from build123d import *

# Parameters (mm, degrees)
SKETCH1_R                                           = 8.5
BOSS_EXTRUDE1_DEPTH                                 = 33.5
SKETCH2_W                                           = 53
SKETCH2_H                                           = 50
CUT_EXTRUDE1_DEPTH                                  = 30
SKETCH3_W                                           = 53
SKETCH3_H                                           = 10
BOSS_EXTRUDE2_DEPTH                                 = 13
FILLET1_R                                           = 15
CSK_FOR_M4_COUNTERSUNK_FLAT_HEAD_SCREW1_D           = 4.3
CSK_FOR_M4_COUNTERSUNK_FLAT_HEAD_SCREW1_CSINK_D     = 9.4
CSK_FOR_M4_COUNTERSUNK_FLAT_HEAD_SCREW1_CSINK_ANGLE = 90
M4_TAPPED_HOLE1_D                                   = 3.3
CHAMFER1_SIZE                                       = 1
M3_TAPPED_HOLE2_D                                   = 2.5
M3_TAPPED_HOLE2_DEPTH                               = 7
M4_TAPPED_HOLE2_D                                   = 3.3
M4_TAPPED_HOLE2_DEPTH                               = 16
M4_TAPPED_HOLE2_TIP                                 = 0.991420021
M4_CLEARANCE_HOLE1_D                                = 4.3


with BuildPart() as part:
    # Sketch1 → Boss-Extrude1 (new, symmetric)
    with BuildSketch(Plane(origin=(0, 0, 0), x_dir=(0, 0, -1), z_dir=(1, 0, 0))):
        with BuildLine():
            Line((-7, 26), (-46.256287113, 14.383463422))
            ThreePointArc((-46.256287113, 14.383463422), (-57, 0), (-46.256287113, -14.383463422))
            Line((-46.256287113, -14.383463422), (-7, -26))
            Line((-7, -26), (0, -26))
            Line((0, -26), (0, 26))
            Line((0, 26), (-7, 26))
        make_face()
        with Locations((-42, 0)):
            Circle(SKETCH1_R, mode=Mode.SUBTRACT)
    extrude(amount=BOSS_EXTRUDE1_DEPTH, both=True)

    # Sketch2 → Cut-Extrude1 (cut, symmetric)
    with BuildSketch(Plane(origin=(0, 0, 0), x_dir=(1, 0, 0), z_dir=(0, 1, 0))):
        with Locations((0, -32)):
            Rectangle(SKETCH2_W, SKETCH2_H)
    extrude(amount=CUT_EXTRUDE1_DEPTH, both=True, mode=Mode.SUBTRACT)

    # Sketch3 → Boss-Extrude2 (add)
    with BuildSketch(Plane.XY.offset(7)):
        Rectangle(SKETCH3_W, SKETCH3_H)
    extrude(amount=BOSS_EXTRUDE2_DEPTH)

    # Fillet1
    fillet1_edges = [part.edges().sort_by_distance(p)[0] for p in [
        (-26.5, 5, 13.5),
        (-26.5, -5, 13.5),
        (26.5, -5, 13.5),
        (26.5, 5, 13.5),
    ]]
    fillet(fillet1_edges, radius=FILLET1_R)

    # CSK for M4 Countersunk Flat Head Screw1 (through all)
    with Locations(Plane(origin=(0, 0, 0), x_dir=(-1, 0, 0), z_dir=(0, 0, -1))):
        with Locations((0, 18.5), (0, -18.5)):
            CounterSinkHole(CSK_FOR_M4_COUNTERSUNK_FLAT_HEAD_SCREW1_D / 2, CSK_FOR_M4_COUNTERSUNK_FLAT_HEAD_SCREW1_CSINK_D / 2, counter_sink_angle=CSK_FOR_M4_COUNTERSUNK_FLAT_HEAD_SCREW1_CSINK_ANGLE)

    # M4 Tapped Hole1 (through all)
    with Locations(Plane.XY.offset(20)):
        with Locations((0, 0)):
            Hole(M4_TAPPED_HOLE1_D / 2)

    # Chamfer1
    chamfer1_edges = [part.edges().sort_by_distance(p)[0] for p in [
        (-33.5, 0, 50.5),
        (33.5, 0, 50.5),
    ]]
    chamfer(chamfer1_edges, length=CHAMFER1_SIZE)

    # M3 Tapped Hole2
    with Locations(Plane(origin=(33.5, 0, 0), x_dir=(0, 0, -1), z_dir=(1, 0, 0))):
        with Locations((-34.221825407, 7.778174593), (-49.778174593, 7.778174593), (-34.221825407, -7.778174593), (-49.778174593, -7.778174593)):
            m3_tapped_hole2 = Hole(M3_TAPPED_HOLE2_D / 2, depth=M3_TAPPED_HOLE2_DEPTH)

    # Mirror1: M3 Tapped Hole2 across plane
    add(m3_tapped_hole2.mirror(Plane(origin=(0, 0, 0), x_dir=(0, 0, 1), z_dir=(1, 0, 0))), mode=Mode.SUBTRACT)

    # M4 Tapped Hole2
    with Locations(Plane(origin=(0, 0, 0), x_dir=(-1, 0, 0), z_dir=(0, 0, -1))):
        with Locations((-30, 20), (-30, -20), (30, 20), (30, -20), (-30, 0), (30, 0)):
            Hole(M4_TAPPED_HOLE2_D / 2, depth=M4_TAPPED_HOLE2_DEPTH)
            with Locations((0, 0, -(M4_TAPPED_HOLE2_DEPTH + M4_TAPPED_HOLE2_TIP / 2))):  # 118° drill point
                Cone(0, M4_TAPPED_HOLE2_D / 2, M4_TAPPED_HOLE2_TIP, mode=Mode.SUBTRACT)

    # M4 Clearance Hole1 (through all)
    with Locations(Plane(origin=(0, 0, 0), x_dir=(-1, 0, 0), z_dir=(0, 0, -1))):
        with Locations((-22.33, 21.75), (22.33, -21.75), (22.33, 21.75), (-22.33, -21.75)):
            Hole(M4_CLEARANCE_HOLE1_D / 2)


solid = part.part
CAD build for the part. Positions are in the model's coordinates, mm. A direction names the side the tool comes from. Round coordinates to 2 decimals unless told otherwise and drop trailing zeros. Order: outer loops, then holes, each group sorted by start corner. A loop starts at its lowest first (then second) coordinate and runs counter-clockwise, first axis right, second up. Notation, with made-up numbers: (78, 69) -> (128, 69) arc R34 ccw to (128, 103) -> close; hole circle Ø5 at (-5.75, -34). An arc over 180 degrees is marked (long way). Write item = value, one per line. Start each with the question number.
(1) Pin check, flat tips, straight feed: P1, Ø4, axis at x = 2, z = 14.5, coming from the +Y side; P2, Ø2.5, axis at x = 0, y = 0, coming from the -Z side; P3, Ø10, axis at x = -1, y = -18.5, coming from the +Z side; P4, Ø5.5, axis at x = 0, y = 18.5, coming from the -Z side. Stop position of each tip, or through.
(2) Pull direction X, two halves, no side cores. Call faces 6 (the flat face through (0, 5, 13)), 7 (the flat face through (33.5, 0, 23)), 8 (the cylindrical face through (-29.95, 8.15, 50.97)): released by +X, released by -X, zero draft, split by the parting line, or undercut.
(3) Cut at C-C, the plane z = 12.5. List the corners of the cut face in (x, y).
(4) Cut at B-B, the plane z = 30.5. List the corners of the cut face in (x, y), then the cut area to 3 significant figures.
(5) Probe line 1 (Y direction, x = 0, z = 6.1); line 2 (X direction, y = 12, z = 24.5); line 3 (Y direction, x = -1, z = 6). List the from-to ranges inside material, lowest first. Write a range as [from, to].
(6) Cut at A-A, the plane x = -23.5. List the corners of the cut face in (y, z).
(7) Which spindle directions (+Z, -Z, +X, -X, +Y, -Y) get a long thin tool onto all of the face, cutting with end or side? Do faces 1 (the flat face through (-29.95, -20.11, 26.9)), 2 (the cylindrical face through (29.458, 5.745, 48.265)), 3 (the cylindrical face through (28.35, 0.07, 8.11)), 4 (the cylindrical face through (21.99, 9.28, 13.59)), 5 (the flat face through (-0.4, 4.7, 20)). Say none if no direction does.
(8) Cut at D-D, the plane z = 42. List the corners of the cut face in (x, y).
Model answer:
q1.P1 = 5
q1.P2 = through
q1.P3 = 7
q1.P4 = 1.95
q2.face_6 = undercut
q2.face_7 = released by +X
q2.face_8 = zero draft
q3.outline = (-33.5, -24.37) -> (-26.5, -24.37) -> (-26.5, -20) arc R15 cw to (-11.5, -5) -> (11.5, -5) arc R15 cw to (26.5, -20) -> (26.5, -24.37) -> (33.5, -24.37) -> (33.5, 24.37) -> (26.5, 24.37) -> (26.5, 20) arc R15 cw to (11.5, 5) -> (-11.5, 5) arc R15 cw to (-26.5, 20) -> (-26.5, 24.37) -> (-33.5, 24.37) -> close; hole circle Ø3.3 at (-30, -20); hole circle Ø3.3 at (-30, 0); hole circle Ø3.3 at (-30, 20); hole circle Ø3.3 at (0, 0); hole circle Ø3.3 at (30, -20); hole circle Ø3.3 at (30, 0); hole circle Ø3.3 at (30, 20)
q4.outline = (-33.5, -19.05) -> (-26.5, -19.05) -> (-26.5, 19.05) -> (-33.5, 19.05) -> close; (26.5, -19.05) -> (33.5, -19.05) -> (33.5, 19.05) -> (26.5, 19.05) -> close
q4.area = 533 mm2
q5.line_1 = [-26, -20.65], [-16.35, -1.65], [1.65, 16.35], [20.65, 26]
q5.line_2 = [-33.5, -26.5], [26.5, 33.5]
q5.line_3 = [-26, -20.4], [-16.6, -1.31], [1.31, 16.6], [20.4, 26]
q6.outline = (-26, 0) -> (-23.55, 0) -> (-23.55, 7) -> (-26, 7) -> close; (-19.95, 0) -> (19.95, 0) -> (19.95, 7) -> (11, 7) -> (11, 20) -> (-11, 20) -> (-11, 7) -> (-19.95, 7) -> close; (23.55, 0) -> (26, 0) -> (26, 7) -> (23.55, 7) -> close
q7.face_1 = +Z, +X, -X, -Y
q7.face_2 = +X, -X
q7.face_3 = -Z
q7.face_4 = +Z, +Y
q7.face_5 = +Z, +Y, -Y
q8.outline = (-33.5, -15.64) -> (-26.5, -15.64) -> (-26.5, -8.5) -> (-32.5, -8.5) -> (-33.5, -9.5) -> close; (-33.5, 9.5) -> (-32.5, 8.5) -> (-26.5, 8.5) -> (-26.5, 15.64) -> (-33.5, 15.64) -> close; (26.5, -15.64) -> (33.5, -15.64) -> (33.5, -9.5) -> (32.5, -8.5) -> (26.5, -8.5) -> close; (26.5, 8.5) -> (32.5, 8.5) -> (33.5, 9.5) -> (33.5, 15.64) -> (26.5, 15.64) -> close
